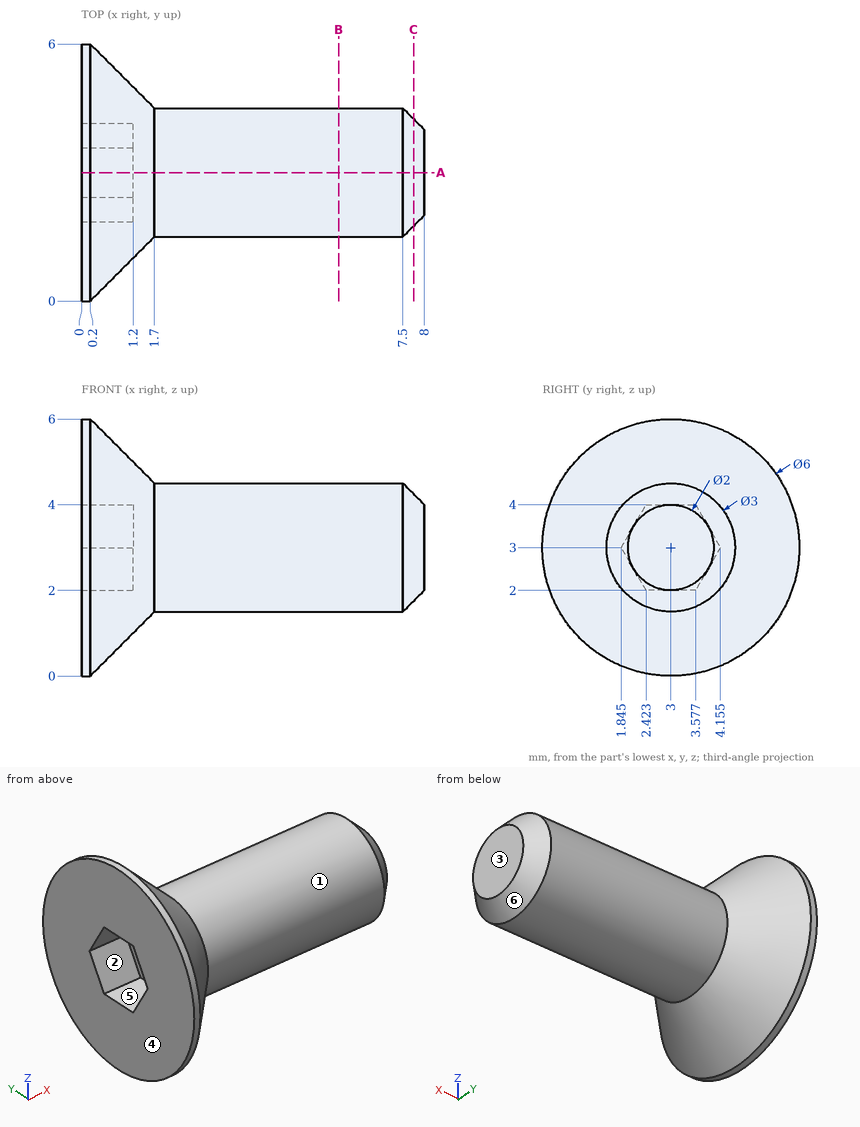
Verification items for this drawing (mm, ordinates from the low corner). A direction names the side the tool comes from. Coordinates: 2 decimals unless noted, no trailing zeros. Write each loop counter-clockwise with the first axis right and the second up, starting at its lowest first coordinate (ties: lowest second). Pieces come first, ordered by that corner, then holes. Notation, with made-up numbers: M 83,0 L 136,0 A27 ccw 136,32 Z; hole C 58.5,-22.5 d10. An arc over 180 degrees is marked long. Answer as a JSON object with one key per item and string values.
1. Scan lines: L1, parallel to X at y = 3.15, z = 2.7; L2, parallel to Y at x = 0.5, z = 2.4; L3, parallel to Z at x = 2, y = 3.55 (1 decimal). Record each from-to range of solid material in increasing order.
Answers below:
{"L1": "x = 1.2 to 8", "L2": "y = 0.37 to 2.19, 3.81 to 5.63", "L3": "z = 1.6 to 4.4"}
2. Draft check along Z on the marked faces 4, 5 and 6. Enter one of: released by +Z, released by -Z, zero draft, split by the parting line, or undercut.
Answers below:
{"face 4": "zero draft", "face 5": "undercut", "face 6": "split by the parting line"}
3. Section check B-B, the plane x = 6. Enter the section's corners in (y, z).
Answers below:
{"outline": "C 3,3 d3"}
4. Go/stop test with flat-tipped pins: pin 1 Ø3 at (x, y) = (2, 1) entering from +Z (1 decimal); pin 2 Ø1.5 at (x, y) = (3.5, 1) entering from -Z; pin 3 Ø1 at (x, z) = (4.5, 4.5) entering from -Y. Record where each tip stops, or that it passes through.
Answers below:
{"pin 1": "stops at z = 5.2", "pin 2": "stops at z = 2.17", "pin 3": "stops at y = 1.88"}
5. Section check C-C, the plane x = 7.75. Enter the section's corners in (y, z).
Answers below:
{"outline": "C 3,3 d2.5"}
6. Section check A-A, the plane y = 3. Enter the section's corners in (x, z).
Answers below:
{"outline": "M 0,0 L 0.2,0 L 1.7,1.5 L 7.5,1.5 L 8,2 L 8,4 L 7.5,4.5 L 1.7,4.5 L 0.2,6 L 0,6 L 0,4 L 1.2,4 L 1.2,2 L 0,2 Z"}
7. Tool access check on the marked faces 1, 2 and 3. Record the directions out of +Z, -Z, +X, -X, +Y, -Y that give a thin tool (end or side, any length) a straight path to the whole face; none if there is none.
Answers below:
{"face 1": "+X", "face 2": "-X", "face 3": "+Z, -Z, +X, +Y, -Y"}
